Can you work these out from the model? Positions are in its coordinate system, mm. Coordinates: 2 decimals unless noted, no trailing zeros. Write each loop counter-clockwise with the first axis right and the second up, starting at its lowest first coordinate (ties: lowest second). Pieces come first, ordered by that corner, then holes. Notation, with made-up numbers: (15, 55.25) - (46, 55.25) arc R23 cw to (46, 91.25) - close; hole circle Ø6 at (-13, 66). An arc over 180 degrees is marked (long way). Write each question's results on one line, items separated by ' | '. Start each with the question number.
```python
from build123d import *

# Parameters (mm, degrees)
SKETCH1_R           = 11
SKETCH1_R_2         = 1.55
BOSS_EXTRUDE1_DEPTH = 2
SKETCH2_R           = 2.05
CUT_EXTRUDE1_DEPTH  = 30.83630339
SKETCH5_W           = 5.3
SKETCH5_H           = 10
BOSS_EXTRUDE3_DEPTH = 2
FILLET1_R           = 2
SKETCH6_R           = 1.5
CUT_EXTRUDE3_DEPTH  = 34.784981871
SKETCH7_R           = 2
CUT_EXTRUDE6_DEPTH  = 34.784981871


with BuildPart() as part:
    # Sketch1 → Boss-Extrude1 (new body)
    with BuildSketch(Plane.XY):
        with BuildLine():
            Line((-21.05, 15.5), (-21.05, -15.5))
            ThreePointArc((-21.05, -15.5), (-19.424442636, -19.424442636), (-15.5, -21.05))
            Line((-15.5, -21.05), (15.5, -21.05))
            ThreePointArc((15.5, -21.05), (19.424442636, -19.424442636), (21.05, -15.5))
            Line((21.05, -15.5), (21.05, 15.5))
            ThreePointArc((21.05, 15.5), (19.424442636, 19.424442636), (15.5, 21.05))
            Line((15.5, 21.05), (-15.5, 21.05))
            ThreePointArc((-15.5, 21.05), (-19.424442636, 19.424442636), (-21.05, 15.5))
        make_face()
        Circle(SKETCH1_R, mode=Mode.SUBTRACT)
        with Locations((-15.5, -15.5)):
            Circle(SKETCH1_R_2, mode=Mode.SUBTRACT)
        with Locations((15.5, 15.5)):
            Circle(SKETCH1_R_2, mode=Mode.SUBTRACT)
        with Locations(Location((-15.5, 15.5, 0), (0, 0, 180))):
            Circle(SKETCH1_R_2, mode=Mode.SUBTRACT)
        with Locations((15.5, -15.5)):
            Circle(SKETCH1_R_2, mode=Mode.SUBTRACT)
    extrude(amount=BOSS_EXTRUDE1_DEPTH)

    # Sketch2 → Cut-Extrude1 (cut, through all)
    with BuildSketch(Plane.XY.offset(2)):
        with Locations((0, -17.5)):
            Circle(SKETCH2_R)
    extrude(amount=-CUT_EXTRUDE1_DEPTH, mode=Mode.SUBTRACT)

    # Sketch5 → Boss-Extrude3 (add)
    with BuildSketch(Plane(origin=(0, 0, 0), x_dir=(-1, 0, 0), z_dir=(0, 0, -1))):
        with Locations((-23.7, -3.5)):
            Rectangle(SKETCH5_W, SKETCH5_H)
    extrude(amount=-BOSS_EXTRUDE3_DEPTH)

    # Fillet1
    fillet1_edges = [part.edges().sort_by_distance(p)[0] for p in [
        (26.35, -8.5, 1),
        (26.35, 1.5, 1),
    ]]
    fillet(fillet1_edges, radius=FILLET1_R)

    # Sketch6 → Cut-Extrude3 (cut, through all)
    with BuildSketch(Plane.XY.offset(2)):
        with Locations((22.110660172, 2.560660172)):
            Circle(SKETCH6_R)
        with Locations((22.110660172, -9.560660172)):
            Circle(SKETCH6_R)
    extrude(amount=-CUT_EXTRUDE3_DEPTH, mode=Mode.SUBTRACT)

    # Sketch7 → Cut-Extrude6 (cut, through all)
    with BuildSketch(Plane(origin=(0, 0, 0), x_dir=(-1, 0, 0), z_dir=(0, 0, -1))):
        with Locations((-13.95, 3.05)):
            Circle(SKETCH7_R)
        with Locations((16.55, -9)):
            Circle(SKETCH7_R)
    extrude(amount=-CUT_EXTRUDE6_DEPTH, mode=Mode.SUBTRACT)


solid = part.part
```
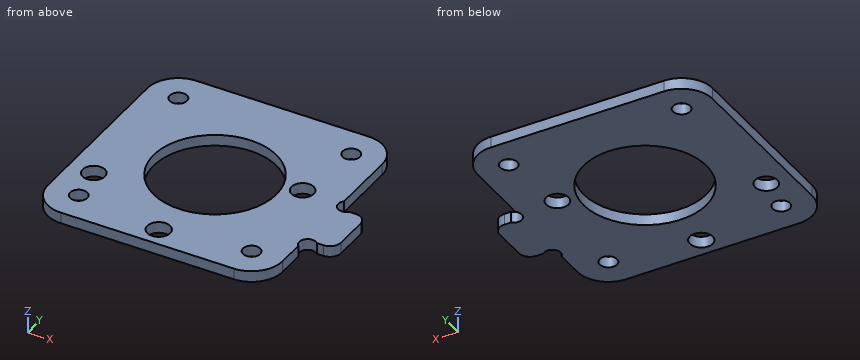
Q1. If we section it at B-B (z = 0.6): Count the separate pieces of the cut face and the enclosed holes in it, then the cut area to 3 significant figures.
Q2. I need wall thicknesses on line 1 along Y through (x, z) = (-16.55, 0.55); line 2 along X through (y, z) = (-10, 1.7); line 3 along X through (y, z) = (-8, 1.3). Which ranges of each line are inside material? Lowest first, please. Write a range as from..to.
Q3. If we section it at C-C (y = 3.05): Please give me the cut outline in (x, z), then the cut area to 3 significant figures.
Q4. If we section it at A-A (x = 0): Please give me the cut outline in (y, z), then the cut area to 3 significant figures.
Q5. If we section it at D-D (x = -10): Please give me the cut outline in (y, z), then the cut area to 3 significant figures.
Answer list:
1) separate pieces: 1 | enclosed holes: 8 | area: 1,350 mm2
2) line 1: y = -20.95..-16.64, -14.36..-11, -7..14.36, 16.64..20.95 | line 2: x = -21.05..-18.28, -14.82..-4.58, 4.58..20.68 | line 3: x = -21.05..-18.28, -14.82..-7.55, 7.55..25.67
3) outline: (-21.05, 0) - (-10.57, 0) - (-10.57, 2) - (-21.05, 2) - close; (10.57, 0) - (11.95, 0) - (11.95, 2) - (10.57, 2) - close; (15.95, 0) - (20.69, 0) - (20.69, 2) - (15.95, 2) - close | area: 33.2 mm2
4) outline: (-21.05, 0) - (-19.55, 0) - (-19.55, 2) - (-21.05, 2) - close; (-15.45, 0) - (-11, 0) - (-11, 2) - (-15.45, 2) - close; (11, 0) - (21.05, 0) - (21.05, 2) - (11, 2) - close | area: 32.0 mm2
5) outline: (-21.05, 0) - (-4.58, 0) - (-4.58, 2) - (-21.05, 2) - close; (4.58, 0) - (21.05, 0) - (21.05, 2) - (4.58, 2) - close | area: 65.9 mm2
